Check sheet for the modelled part. Datum: model origin and axes. Units: mm. A direction names the side the tool comes from. Round coordinates to 2 decimals unless told otherwise and drop trailing zeros. Order: outer loops, then holes, each group sorted by start corner. A loop starts at its lowest first (then second) coordinate and runs counter-clockwise, first axis right, second up.
(1) Thickness scan on probe 1 along X at (y, z) = (67.5, 13); probe 2 along X at (y, z) = (105, 14); probe 3 along X at (y, z) = (-35, 6). Record the ranges inside material, lowest first.
(2) Sectioned sample at A-A, the plane x = 82.5. Enter the section's corners in (y, z).
(3) Tool access check on faces 4 (the flat face through (92.323, -74.175, 9.392)), 5 (the flat face through (108, -9, 19.05)). Record the directions out of +Z, -Z, +X, -X, +Y, -Y that give a thin tool (end or side, any length) a straight path to the whole face; none if there is none.
(4) Mould release check, pull along X, two halves, no side actions. Record for faces 1 (the cylindrical face through (2.476, -147.963, 9.658)), 2 (the flat face through (187.44, 86.7, 9.66)), 3 (the flat face through (114.66, 66.2, 9.39)): released by +X, released by -X, zero draft, split by the parting line, or undercut.
(5) Depth check by flat-ended pin: pin 1 (5 mm diameter, centred on x = 59, z = 6.5, fed in from -Y); pin 2 (4 mm diameter, centred on y = -41.5, z = 12.5, fed in from +X); pin 3 (4 mm diameter, centred on y = -32, z = 13, fed in from +X). Enter the tip coordinate at first touch or a pass-through.
(6) Sectioned sample at B-B, the plane z = 15.25. Count the separate pieces of the cut face and the enclosed holes in it, and give its area (3 significant figures).
```python
from build123d import *

# Parameters (mm, degrees)
F2_DEPTH = 19.05
F3_DEPTH = 25.4
F5_DEPTH = 25.4
F6_R     = 12.7
F7_R     = 5.08


with BuildPart() as f2:
    # F0 (on Top) → F2 (new body)
    with BuildSketch(Plane.XY):
        Polygon((219.970453, 127), (0, 0), (0, -152.4), (219.970453, -25.4), align=None)
    extrude(amount=F2_DEPTH)

    # F1 (on face) → F3 (cut)
    with BuildSketch(Plane.XY):
        Polygon((148.085226, 56.167652), (38.1, -7.332348), (38.1, -17.492348), (148.085226, 46.007652), align=None)
        Polygon((38.1, -105.480529), (148.085226, -41.980529), (148.085226, -31.820529), (38.1, -95.320529), align=None)
    extrude(amount=F3_DEPTH, mode=Mode.SUBTRACT)

    # F4 (on face) → F5 (cut)
    with BuildSketch(Plane.XY.offset(19.05)):
        Polygon((219.970453, 119.667652), (219.970453, 123.333826), (153.979317, 85.233826), (153.979317, 81.567652), align=None)
        Polygon((219.970453, 114.407963), (153.979317, 76.307963), (153.979317, 72.641788), (219.970453, 110.741788), align=None)
        Polygon((219.970453, 105.4821), (153.979317, 67.3821), (153.979317, 63.715925), (219.970453, 101.815925), align=None)
        Polygon((219.970453, 96.556236), (153.979317, 58.456236), (153.979317, 54.790062), (219.970453, 92.890062), align=None)
        Polygon((219.970453, 87.630373), (153.979317, 49.530373), (153.979317, 45.864199), (219.970453, 83.964199), align=None)
        Polygon((219.970453, 78.70451), (153.979317, 40.60451), (153.979317, 36.938336), (219.970453, 75.038336), align=None)
        Polygon((219.970453, 69.778647), (153.979317, 31.678647), (153.979317, 28.012473), (219.970453, 66.112473), align=None)
        Polygon((219.970453, 60.852784), (153.979317, 22.752784), (153.979317, 19.08661), (219.970453, 57.18661), align=None)
        Polygon((219.970453, 51.926921), (153.979317, 13.826921), (153.979317, 10.160747), (219.970453, 48.260747), align=None)
        Polygon((219.970453, 43.001058), (153.979317, 4.901058), (153.979317, 1.234883), (219.970453, 39.334883), align=None)
        Polygon((219.970453, 34.075195), (153.979317, -4.024805), (153.979317, -7.69098), (219.970453, 30.40902), align=None)
        Polygon((219.970453, 25.149331), (153.979317, -12.950669), (153.979317, -16.616843), (219.970453, 21.483157), align=None)
        Polygon((219.970453, 16.223468), (153.979317, -21.876532), (153.979317, -25.542706), (219.970453, 12.557294), align=None)
        Polygon((219.970453, 7.297605), (153.979317, -30.802395), (153.979317, -34.468569), (219.970453, 3.631431), align=None)
        Polygon((219.970453, -1.628258), (153.979317, -39.728258), (153.979317, -43.394432), (219.970453, -5.294432), align=None)
        Polygon((219.970453, -10.554121), (153.979317, -48.654121), (153.979317, -52.320295), (219.970453, -14.220295), align=None)
        Polygon((219.970453, -19.479984), (153.979317, -57.579984), (153.979317, -61.246158), (219.970453, -23.146158), align=None)
        Polygon((219.970453, -28.405847), (153.979317, -66.505847), (153.979317, -70.172022), (219.970453, -32.072022), align=None)
        Polygon((219.970453, -37.33171), (153.979317, -75.43171), (153.979317, -79.097885), (219.970453, -40.997885), align=None)
    extrude(amount=-F5_DEPTH, mode=Mode.SUBTRACT)

    # F6
    f6_edges = [f2.edges().sort_by_distance(p)[0] for p in [
        (0, 0, 9.525),
    ]]
    fillet(f6_edges, radius=F6_R)

    # F7
    f7_edges = [f2.edges().sort_by_distance(p)[0] for p in [
        (0, -152.4, 9.525),
    ]]
    fillet(f7_edges, radius=F7_R)


solid = f2.part
```
Derived:
1. probe 1: x = 116.91 to 154.18, 160.53 to 169.64, 175.99 to 185.1, 191.45 to 200.56, 206.91 to 216.02
1. probe 2: x = 181.87 to 188.22, 194.57 to 203.68, 210.03 to 219.14
1. probe 3: x = 0 to 142.58, 148.09 to 162.17, 168.52 to 177.63, 183.98 to 193.09, 199.44 to 203.34
2. outline: (-104.77, 0) - (-79.85, 0) - (-79.85, 19.05) - (-104.77, 19.05) - close; (-69.69, 0) - (8.14, 0) - (8.14, 19.05) - (-69.69, 19.05) - close; (18.3, 0) - (47.63, 0) - (47.63, 19.05) - (18.3, 19.05) - close
3. face 4: +Z, -Z
3. face 5: +Z, +X, -X, +Y, -Y
4. face 1: split by the parting line
4. face 2: undercut
4. face 3: released by -X
5. pin 1: stops at y = -119.78
5. pin 2: stops at x = 195.55
5. pin 3: stops at x = 212
6. separate pieces: 1
6. enclosed holes: 2
6. area: 27,100 mm2
